```python
from build123d import *

# Parameters (mm, degrees)
SPUR_START             = -16.129320455
SPUR_GEAR_AI_OUTLINE_R = 3.175
SPUR_GEAR_AI_DEPTH     = 5.08
SCALE1_SCALE           = 15


# Read off the part's stored shape, not the designer's step: spur gear_ai
with BuildPart() as part:
    # spur gear_ai outline → spur gear_ai (new body)
    with BuildSketch(Plane.YZ.offset(SPUR_START)):
        with BuildLine():
            ThreePointArc((3.217647432, 17.980210444), (2.945962103, 18.012251215), (2.673552099, 18.037397168))
            ThreePointArc((2.673552099, 18.037397168), (1.882282705, 16.734209467), (1.665300635, 15.22512888))
            ThreePointArc((1.665300635, 15.22512888), (0.986555153, 15.183035327), (0.313890146, 15.083089914))
            ThreePointArc((0.313890146, 15.083089914), (-0.212105842, 16.514080361), (-1.257032059, 17.624276126))
            ThreePointArc((-1.257032059, 17.624276126), (-1.518261113, 17.543042448), (-1.777347815, 17.455215289))
            ThreePointArc((-1.777347815, 17.455215289), (-1.970154185, 15.942855827), (-1.554578797, 14.475987553))
            ThreePointArc((-1.554578797, 14.475987553), (-2.157522658, 14.161462519), (-2.731381258, 13.796560335))
            ThreePointArc((-2.731381258, 13.796560335), (-3.793938754, 14.889893315), (-5.200083652, 15.479097832))
            ThreePointArc((-5.200083652, 15.479097832), (-5.405687554, 15.298635745), (-5.60665251, 15.113021587))
            ThreePointArc((-5.60665251, 15.113021587), (-5.167657883, 13.652991056), (-4.191381798, 12.481969945))
            ThreePointArc((-4.191381798, 12.481969945), (-4.614269567, 11.949397667), (-4.990096395, 11.382633613))
            ThreePointArc((-4.990096395, 11.382633613), (-6.405489555, 11.949261922), (-7.929717906, 11.915596376))
            ThreePointArc((-7.929717906, 11.915596376), (-8.044145874, 11.667109416), (-8.152240417, 11.415802634))
            ThreePointArc((-8.152240417, 11.415802634), (-7.157350952, 10.260553574), (-5.789181173, 9.587859815))
            ThreePointArc((-5.789181173, 9.587859815), (-5.958891714, 8.929326879), (-6.071702896, 8.25869961))
            ThreePointArc((-6.071702896, 8.25869961), (-7.595197385, 8.200648065), (-8.973956261, 7.549933535))
            ThreePointArc((-8.973956261, 7.549933535), (-8.977422659, 7.276387354), (-8.973956261, 7.002841173))
            ThreePointArc((-8.973956261, 7.002841173), (-7.595197384, 6.352126644), (-6.071702896, 6.294075099))
            ThreePointArc((-6.071702896, 6.294075099), (-5.958891714, 5.62344783), (-5.789181173, 4.964914893))
            ThreePointArc((-5.789181173, 4.964914893), (-7.157350952, 4.292221134), (-8.152240417, 3.136972074))
            ThreePointArc((-8.152240417, 3.136972074), (-8.044145874, 2.885665292), (-7.929717906, 2.637178332))
            ThreePointArc((-7.929717906, 2.637178332), (-6.405489555, 2.603512786), (-4.990096395, 3.170141095))
            ThreePointArc((-4.990096395, 3.170141095), (-4.614269567, 2.603377042), (-4.191381798, 2.070804764))
            ThreePointArc((-4.191381798, 2.070804764), (-5.167657883, 0.899783653), (-5.60665251, -0.560246879))
            ThreePointArc((-5.60665251, -0.560246879), (-5.405687554, -0.745861037), (-5.200083652, -0.926323123))
            ThreePointArc((-5.200083652, -0.926323123), (-3.793938754, -0.337118607), (-2.731381258, 0.756214373))
            ThreePointArc((-2.731381258, 0.756214373), (-2.157522658, 0.391312189), (-1.554578797, 0.076787156))
            ThreePointArc((-1.554578797, 0.076787156), (-1.970154185, -1.390081118), (-1.777347815, -2.90244058))
            ThreePointArc((-1.777347815, -2.90244058), (-1.518261113, -2.990267739), (-1.257032059, -3.071501418))
            ThreePointArc((-1.257032059, -3.071501418), (-0.212105842, -1.961305652), (0.313890146, -0.530315206))
            ThreePointArc((0.313890146, -0.530315206), (0.986555153, -0.630260618), (1.665300635, -0.672354172))
            ThreePointArc((1.665300635, -0.672354172), (1.882282705, -2.181434759), (2.673552099, -3.48462246))
            ThreePointArc((2.673552099, -3.48462246), (2.945962103, -3.459476506), (3.217647432, -3.427435736))
            ThreePointArc((3.217647432, -3.427435736), (3.720677732, -1.988211655), (3.619162727, -0.466994991))
            ThreePointArc((3.619162727, -0.466994991), (4.27432425, -0.284702162), (4.911510093, -0.047085877))
            ThreePointArc((4.911510093, -0.047085877), (5.723531449, -1.337445034), (6.976446201, -2.206127982))
            ThreePointArc((6.976446201, -2.206127982), (7.215077342, -2.07235688), (7.450242085, -1.932581801))
            ThreePointArc((7.450242085, -1.932581801), (7.324397959, -0.413184324), (6.612924828, 0.935226378))
            ThreePointArc((6.612924828, 0.935226378), (7.137299488, 1.368237363), (7.62275047, 1.844477471))
            ThreePointArc((7.62275047, 1.844477471), (8.889405244, 0.995954565), (10.38732501, 0.711979544))
            ThreePointArc((10.38732501, 0.711979544), (10.550915796, 0.931245556), (10.708897832, 1.154586562))
            ThreePointArc((10.708897832, 1.154586562), (9.975938874, 2.491439809), (8.777527784, 3.433892087))
            ThreePointArc((8.777527784, 3.433892087), (9.080446439, 4.042749694), (9.330223676, 4.675267385))
            ThreePointArc((9.330223676, 4.675267385), (10.832495749, 4.415298049), (12.316416594, 4.765132816))
            ThreePointArc((12.316416594, 4.765132816), (12.376680691, 5.031980652), (12.430163492, 5.300269897))
            ThreePointArc((12.430163492, 5.300269897), (11.216824963, 6.223424842), (9.73869208, 6.596960136))
            ThreePointArc((9.73869208, 6.596960136), (9.767777341, 7.276387354), (9.73869208, 7.955814572))
            ThreePointArc((9.73869208, 7.955814572), (11.216824963, 8.329349866), (12.430163492, 9.252504811))
            ThreePointArc((12.430163492, 9.252504811), (12.376680691, 9.520794056), (12.316416594, 9.787641893))
            ThreePointArc((12.316416594, 9.787641893), (10.832495749, 10.137476659), (9.330223676, 9.877507324))
            ThreePointArc((9.330223676, 9.877507324), (9.080446439, 10.510025014), (8.777527784, 11.118882621))
            ThreePointArc((8.777527784, 11.118882621), (9.975938874, 12.061334899), (10.708897832, 13.398188146))
            ThreePointArc((10.708897832, 13.398188146), (10.550915796, 13.621529153), (10.38732501, 13.840795164))
            ThreePointArc((10.38732501, 13.840795164), (8.889405244, 13.556820143), (7.62275047, 12.708297238))
            ThreePointArc((7.62275047, 12.708297238), (7.137299488, 13.184537346), (6.612924828, 13.61754833))
            ThreePointArc((6.612924828, 13.61754833), (7.324397959, 14.965959032), (7.450242085, 16.485356509))
            ThreePointArc((7.450242085, 16.485356509), (7.215077342, 16.625131588), (6.976446201, 16.75890269))
            ThreePointArc((6.976446201, 16.75890269), (5.723531449, 15.890219742), (4.911510093, 14.599860585))
            ThreePointArc((4.911510093, 14.599860585), (4.27432425, 14.83747687), (3.619162727, 15.019769699))
            ThreePointArc((3.619162727, 15.019769699), (3.720677732, 16.540986364), (3.217647432, 17.980210444))
        make_face()
        with Locations((1.817577341, 7.276387354)):
            Circle(SPUR_GEAR_AI_OUTLINE_R, mode=Mode.SUBTRACT)
    extrude(amount=SPUR_GEAR_AI_DEPTH)


with BuildPart() as part_1:
    # Scale1: scaled about (-13.589320455, 1.817577341, 7.276387354)
    add(part.part.scale(SCALE1_SCALE).moved(Location((190.25048637, -25.446082774, -101.869422956))))


solid = part_1.part
```
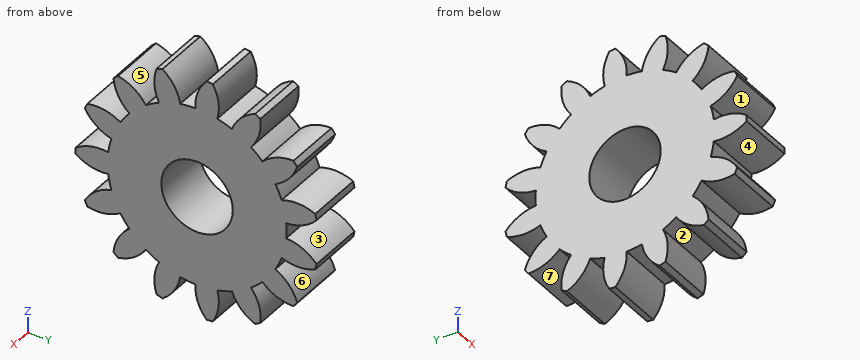
The listing builds one solid part. Answer for the finished solid, in the listing's coordinates (mm). Face numbers are marked on the shaded views. A direction names the side the tool comes from. Coordinates: 2 decimals unless noted, no trailing zeros. Order: outer loops, then holes, each group sorted by start corner. A loop starts at its lowest first (then second) coordinate and runs counter-clockwise, first axis right, second up. Notation, with made-up numbers: M 0,-29 L 52,-29 A18 cw 52,-16 Z; hole C 47.5,47 d3. An arc over 180 degrees is marked long. Answer as a JSON object with one key per item and string values. Group by question number.
1. Section A-A on y = -127 is taken. Write down the section's boundary in (x, z), then the cut area to 3 significant figures.
2. Flat-ended cylindrical pins translate along their axes: P1, Ø5, axis at x = -5.5, y = -94.5, coming from the +Z side; P2, Ø1, axis at x = -12.5, z = 132.5, coming from the +Y side; P3, Ø4, axis at x = -11, z = -100.5, coming from the +Y side. Find the tip coordinate at first contact, or state that the pin passes through.
3. Section B-B on z = 137 is taken. Write down the section's boundary in (x, y).
4. Straight lines are drawn through the part: line 1 (Y direction, x = -28.5, z = 143); line 2 (Z direction, x = 8.5, y = -91); line 3 (Z direction, x = -41, y = -117.5). For each, find the intervals that lie inside material, in ascending order.
5. Section C-C on y = -15.5 is taken. Write down the section's boundary in (x, z), then the cut area to 3 significant figures.
6. Determine the mould class of the marked faces 1, 2 and 3 for opening direction Y: released by +Y, released by -Y, zero draft, split by the parting line, or undercut.
7. A tool of negligible diameter and unlimited length cuts with its end or side. For the marked faces 4, 5, 6 and 7, from which of +Z, -Z, +X, -X, +Y, -Y can it reach the whole face along a straight path? Write none if from no direction.
Values follow:
{
 "1": {"outline": "M -51.69,-63.54 L 24.51,-63.54 L 24.51,-33.54 L -51.69,-33.54 Z; M -51.69,-8.21 L 24.51,-8.21 L 24.51,22.76 L -51.69,22.76 Z; M -51.69,48.09 L 24.51,48.09 L 24.51,78.09 L -51.69,78.09 Z", "area": "6,930 mm2"},
 "2": {"P1": "z = 128.65", "P2": "y = 86.43", "P3": "y = 82.48"},
 "3": {"outline": "M -51.69,-54.98 L 24.51,-54.98 L 24.51,-24.17 L -51.69,-24.17 Z; M -51.69,-0.12 L 24.51,-0.12 L 24.51,30.86 L -51.69,30.86 Z; M -51.69,60.91 L 24.51,60.91 L 24.51,86.69 L -51.69,86.69 Z"},
 "4": {"line 1": "-55.14 to -26.98, 0.97 to 30.71, 67.82 to 86.54", "line 2": "-111.78 to -73.09, -67.6 to 82.15, 87.64 to 126.33", "line 3": "-61.94 to -29.03, -7.61 to 22.16, 43.58 to 76.49"},
 "5": {"outline": "M -51.69,-110.71 L 24.51,-110.71 L 24.51,-37.09 L -51.69,-37.09 Z; M -51.69,51.64 L 24.51,51.64 L 24.51,125.27 L -51.69,125.27 Z", "area": "11,200 mm2"},
 "6": {"face 1": "released by -Y", "face 2": "undercut", "face 3": "released by +Y"},
 "7": {"face 4": "+X, -X", "face 5": "+Z, +X, -X", "face 6": "+X, -X, +Y", "face 7": "-Z, +X, -X"}
}
